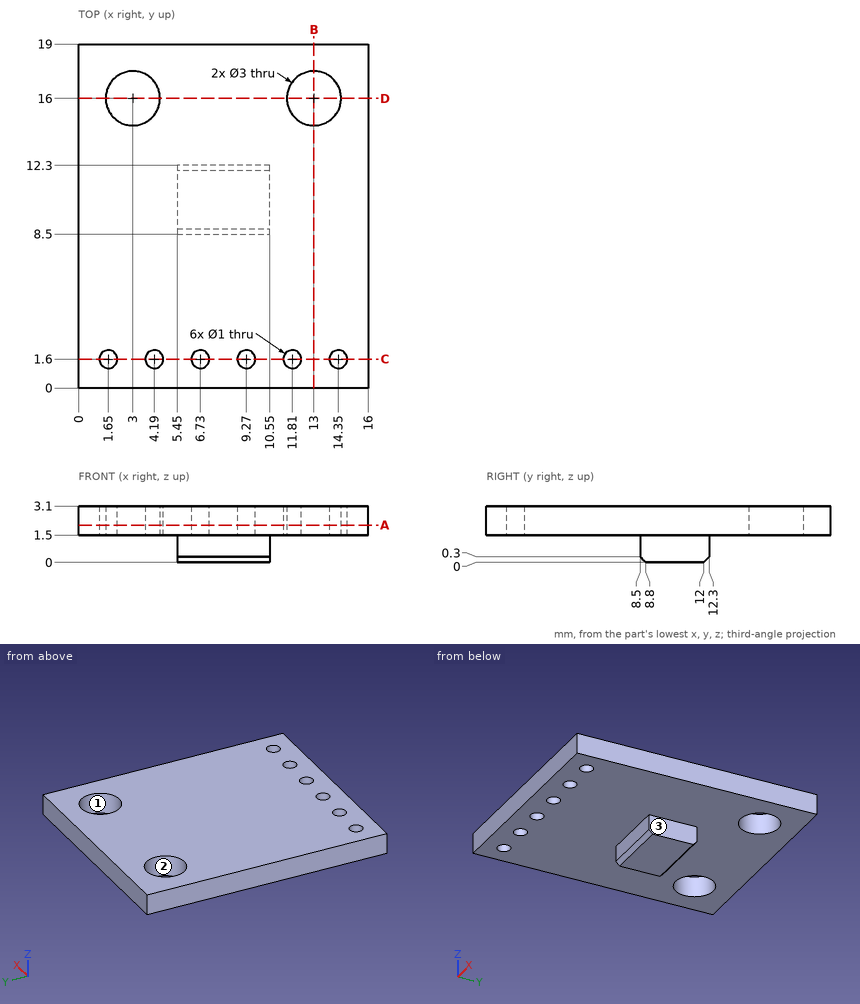
Job drawing, mm, ordinate dimensions from the low corner. One solid piece. Round coordinates to 2 decimals unless told otherwise and drop trailing zeros. Write each loop counter-clockwise with the first axis right and the second up, starting at its lowest first coordinate (ties: lowest second). Pieces come first, ordered by that corner, then holes. Notation, with made-up numbers: (-35.75, -38.5) -> (13.25, -38.5) arc R21 ccw to (13.25, -31.5) -> close; hole circle Ø6 at (-29, 32.5). An arc over 180 degrees is marked (long way). Answer as CSV lines item,"result".
1. Slice it at C-C, the plane y = 1.6. List the corners of the cut face in (x, z).
Resolved:
outline,"(0, 1.5) -> (1.15, 1.5) -> (1.15, 3.1) -> (0, 3.1) -> close; (2.15, 1.5) -> (3.69, 1.5) -> (3.69, 3.1) -> (2.15, 3.1) -> close; (4.69, 1.5) -> (6.23, 1.5) -> (6.23, 3.1) -> (4.69, 3.1) -> close; (7.23, 1.5) -> (8.77, 1.5) -> (8.77, 3.1) -> (7.23, 3.1) -> close; (9.77, 1.5) -> (11.31, 1.5) -> (11.31, 3.1) -> (9.77, 3.1) -> close; (12.31, 1.5) -> (13.85, 1.5) -> (13.85, 3.1) -> (12.31, 3.1) -> close; (14.85, 1.5) -> (16, 1.5) -> (16, 3.1) -> (14.85, 3.1) -> close"
2. Slice it at D-D, the plane y = 16. List the corners of the cut face in (x, z).
Resolved:
outline,"(0, 1.5) -> (1.5, 1.5) -> (1.5, 3.1) -> (0, 3.1) -> close; (4.5, 1.5) -> (11.5, 1.5) -> (11.5, 3.1) -> (4.5, 3.1) -> close; (14.5, 1.5) -> (16, 1.5) -> (16, 3.1) -> (14.5, 3.1) -> close"
3. Slice it at B-B, the plane x = 13. List the corners of the cut face in (y, z).
Resolved:
outline,"(0, 1.5) -> (14.5, 1.5) -> (14.5, 3.1) -> (0, 3.1) -> close; (17.5, 1.5) -> (19, 1.5) -> (19, 3.1) -> (17.5, 3.1) -> close"
4. Drill centre lines: line 1 (Z direction, x = 8.25, y = 12.5); line 2 (Y direction, x = 7, z = 1.25); line 3 (Y direction, x = 4.19, z = 2.4). Where is each one in solid material? Low to high.
Resolved:
line 1,"1.5 to 3.1"
line 2,"8.5 to 12.3"
line 3,"0 to 1.1, 2.1 to 15.09, 16.91 to 19"
5. Mould opens along Y. For the marked faces 1, 2 and 3 say: +Y half, -Y half, draft (parallel to the pull), parting line (faces both ways), or undercut.
Resolved:
face 1,"undercut"
face 2,"undercut"
face 3,"draft"
6. Slice it at A-A, the plane z = 2.05. State how many separate pieces and enclosed holes the cut face has, plus the area to 3 significant figures.
Resolved:
separate pieces,"1"
enclosed holes,"8"
area,"285 mm²"
7. Pin check, flat tips, straight feed: pin 1 Ø1.2 at (y, z) = (9.5, 0.5) entering from -X; pin 2 Ø0.8 at (y, z) = (11.5, 0.5) entering from +X; pin 3 Ø0.6 at (x, z) = (7, 1) entering from -Y. Stop position of each tip, or through.
Resolved:
pin 1,"x = 5.45"
pin 2,"x = 10.55"
pin 3,"y = 8.5"
